Geometry check sheet. Reference: the model listing, model coordinates, mm. A direction names the side the tool comes from. Coordinates: 2 decimals unless noted, no trailing zeros. Write each loop counter-clockwise with the first axis right and the second up, starting at its lowest first coordinate (ties: lowest second). Pieces come first, ordered by that corner, then holes. Notation, with made-up numbers: (66.25, 47) -> (115.25, 47) arc R18 cw to (115.25, 82) -> close; hole circle Ø10 at (37, 33). An arc over 180 degrees is marked (long way). Use a Markdown table: item, result.
```python
from build123d import *

# Parameters (mm, degrees)
ESBO_O1_R                = 1.465754988
RESSALTO_EXTRUS_O1_DEPTH = 1.75
ESBO_O2_W                = 2
ESBO_O2_H                = 2
RESSALTO_EXTRUS_O2_DEPTH = 2.5
FILETE1_R                = 10


with BuildPart() as part:
    # Esboço1 → Ressalto-extrusão1 (new body)
    with BuildSketch(Plane(origin=(0, 0, 0), x_dir=(0, 1, 0), z_dir=(0, 0, 1))):
        with BuildLine():
            Line((3.378557636, 38.25), (11.5, 38.25))
            Line((11.5, 38.25), (11.5, -38.25))
            Line((11.5, -38.25), (-11.5, -38.25))
            Line((-11.5, -38.25), (-11.5, 38.25))
            Line((-11.5, 38.25), (-3.378557636, 38.25))
            Line((-3.378557636, 38.25), (-3.378557636, 43.5))
            ThreePointArc((-3.378557636, 43.5), (0, 46.878557636), (3.378557636, 43.5))
            Line((3.378557636, 43.5), (3.378557636, 38.25))
        make_face()
        with Locations(Location((0, 43.5, 0), (0, 0, 270))):
            Circle(ESBO_O1_R, mode=Mode.SUBTRACT)
    extrude(amount=RESSALTO_EXTRUS_O1_DEPTH)

    # Esboço2 → Ressalto-extrusão2 (add)
    with BuildSketch(Plane(origin=(38.25, 0, 0), x_dir=(0, 0, -1), z_dir=(1, 0, 0))):
        with Locations((-2.74, -5)):
            Rectangle(ESBO_O2_W, ESBO_O2_H)
        with Locations((-2.74, 5)):
            Rectangle(ESBO_O2_W, ESBO_O2_H)
    extrude(amount=RESSALTO_EXTRUS_O2_DEPTH)

    # Filete1
    # the kernel refuses this fillet: 10 mm, written as the material it adds along each edge
    with BuildSketch(Plane(origin=(38.25, 10.966608667, 1.75), x_dir=(-1, 0, 0), z_dir=(0, -1, 0))) as filete1_piece_1_section:
        with BuildLine():
            CenterArc((5.986643467, -10), FILETE1_R, 90, 36.774298296)
            Line((0, -1.99), (0, 0))
            Line((0, 0), (5.986643467, 0))
        make_face()
    filete1_piece_1 = extrude(amount=31.933217335, mode=Mode.PRIVATE)
    filete1_piece_1 = split(filete1_piece_1, bisect_by=Plane(origin=(35.424027316, 4, 2.241553218), z_dir=(0, 1, 0)), keep=Keep.TOP, mode=Mode.PRIVATE)
    filete1_piece_1 = split(filete1_piece_1, bisect_by=Plane(origin=(35.424027316, 6, 2.241553218), z_dir=(0, -1, 0)), keep=Keep.TOP, mode=Mode.PRIVATE)
    add(filete1_piece_1)
    with BuildSketch(Plane(origin=(38.25, -4, 1.75), x_dir=(-1, 0, 0), z_dir=(0, -1, 0)), Plane(origin=(38.25, 6, 1.75), x_dir=(-1, 0, 0), z_dir=(0, -1, 0))) as filete1_piece_2:
        with BuildLine():
            CenterArc((5.986643467, -10), FILETE1_R, 90, 36.774298296)
            Line((0, -1.99), (0, 0))
            Line((0, 0), (5.986643467, 0))
        make_face()
    extrude(amount=2)
    with BuildSketch(Plane(origin=(38.25, 20.966608667, 1.75), x_dir=(-1, 0, 0), z_dir=(0, -1, 0))) as filete1_piece_3_section:
        with BuildLine():
            CenterArc((5.986643467, -10), FILETE1_R, 90, 36.774298296)
            Line((0, -1.99), (0, 0))
            Line((0, 0), (5.986643467, 0))
        make_face()
    filete1_piece_3 = extrude(amount=31.933217335, mode=Mode.PRIVATE)
    filete1_piece_3 = split(filete1_piece_3, bisect_by=Plane(origin=(35.424027316, -6, 2.241553218), z_dir=(0, 1, 0)), keep=Keep.TOP, mode=Mode.PRIVATE)
    filete1_piece_3 = split(filete1_piece_3, bisect_by=Plane(origin=(35.424027316, -4, 2.241553218), z_dir=(0, -1, 0)), keep=Keep.TOP, mode=Mode.PRIVATE)
    add(filete1_piece_3)


solid = part.part
```
Item 1: Section check D-D on x = 12.5. Record the boundary of the cut face in (y, z).
Answer block:
| item | result |
|---|---|
| outline | (-11.5, 0) -> (11.5, 0) -> (11.5, 1.75) -> (-11.5, 1.75) -> close |
Item 2: Mould release check, pull along Y, two halves, no side actions. Record for faces 1 (the flat face through (39, 5, 3.74)), 2 (the flat face through (1, -11.5, 1)), 3 (the cylindrical face through (-42.146, -0.561, 0.863)): +Y half, -Y half, draft (parallel to the pull), parting line (faces both ways), or undercut.
Answer block:
| item | result |
|---|---|
| face 1 | draft |
| face 2 | -Y half |
| face 3 | undercut |
Item 3: Section check A-A on y = 0. Record the boundary of the cut face in (x, z), then the cut area to 3 significant figures.
Answer block:
| item | result |
|---|---|
| outline | (-46.88, 0) -> (-44.97, 0) -> (-44.97, 1.75) -> (-46.88, 1.75) -> close; (-42.03, 0) -> (38.25, 0) -> (38.25, 1.75) -> (-42.03, 1.75) -> close |
| area | 144 mm^2 |
Item 4: Thickness scan on L1, parallel to Y at x = -43.5, z = 0.5; L2, parallel to X at y = -7, z = 1.25; L3, parallel to Z at x = -10, y = -10. Record the ranges inside material, lowest first. Write a range as [from, to].
Answer block:
| item | result |
|---|---|
| L1 | y = [-3.38, -1.47], [1.47, 3.38] |
| L2 | x = [-38.25, 38.25] |
| L3 | z = [0, 1.75] |
Item 5: Tool access check on faces 4 (the flat face through (-41, 3.379, 1)), 5 (the flat face through (-41, -3.379, 1)), 6 (the flat face through (39, 5, 1.74)). Record the directions out of +Z, -Z, +X, -X, +Y, -Y that give a thin tool (end or side, any length) a straight path to the whole face; none if there is none.
Answer block:
| item | result |
|---|---|
| face 4 | +Z, -Z, -X, +Y |
| face 5 | +Z, -Z, -X, -Y |
| face 6 | -Z, +X, +Y, -Y |
Item 6: Section check B-B on z = 2.6. Record the boundary of the cut face in (x, y), then the cut area to 3 significant figures.
Answer block:
| item | result |
|---|---|
| outline | (36.3, -6) -> (40.75, -6) -> (40.75, -4) -> (36.3, -4) -> close; (36.3, 4) -> (40.75, 4) -> (40.75, 6) -> (36.3, 6) -> close |
| area | 17.8 mm^2 |
Item 7: Depth check by flat-ended pin: P1, Ø12, axis at x = -11.5, y = 7.5, coming from the +Z side; P2, Ø1.4, axis at y = 7, z = 0.5, coming from the -X side; P3, Ø1.8, axis at x = -43.5, y = 0, coming from the -Z side; P4, Ø1.6, axis at x = 39.5, y = -5, coming from the -Z side. Enter the tip coordinate at first touch or a pass-through.
Answer block:
| item | result |
|---|---|
| P1 | stops at z = 1.75 |
| P2 | stops at x = -38.25 |
| P3 | passes through |
| P4 | stops at z = 1.74 |
Item 8: Section check C-C on y = -5. Record the boundary of the cut face in (x, z), then the cut area to 3 significant figures.
Answer block:
| item | result |
|---|---|
| outline | (-38.25, 0) -> (38.25, 0) -> (38.25, 1.74) -> (40.75, 1.74) -> (40.75, 3.74) -> (38.25, 3.74) arc R10 cw to (32.26, 1.75) -> (-38.25, 1.75) -> close |
| area | 143 mm^2 |
